Could you check a few things on this drawing? It's one solid part, dimensions in mm from its lowest x, y, z. A direction names the side the tool comes from. Round coordinates to 2 decimals unless told otherwise and drop trailing zeros. Loops run counter-clockwise (first coordinate to the right, second up) from the corner with the lowest first, then second, coordinate; pieces in that order, holes last. Notation, with made-up numbers: M 26,-1.75 L 31,-1.75 A11 ccw 31,7.25 Z; hole C 32.25,-27 d3. An arc over 180 degrees is marked long. Put each result on its own line as item: value. Start each with the question number.
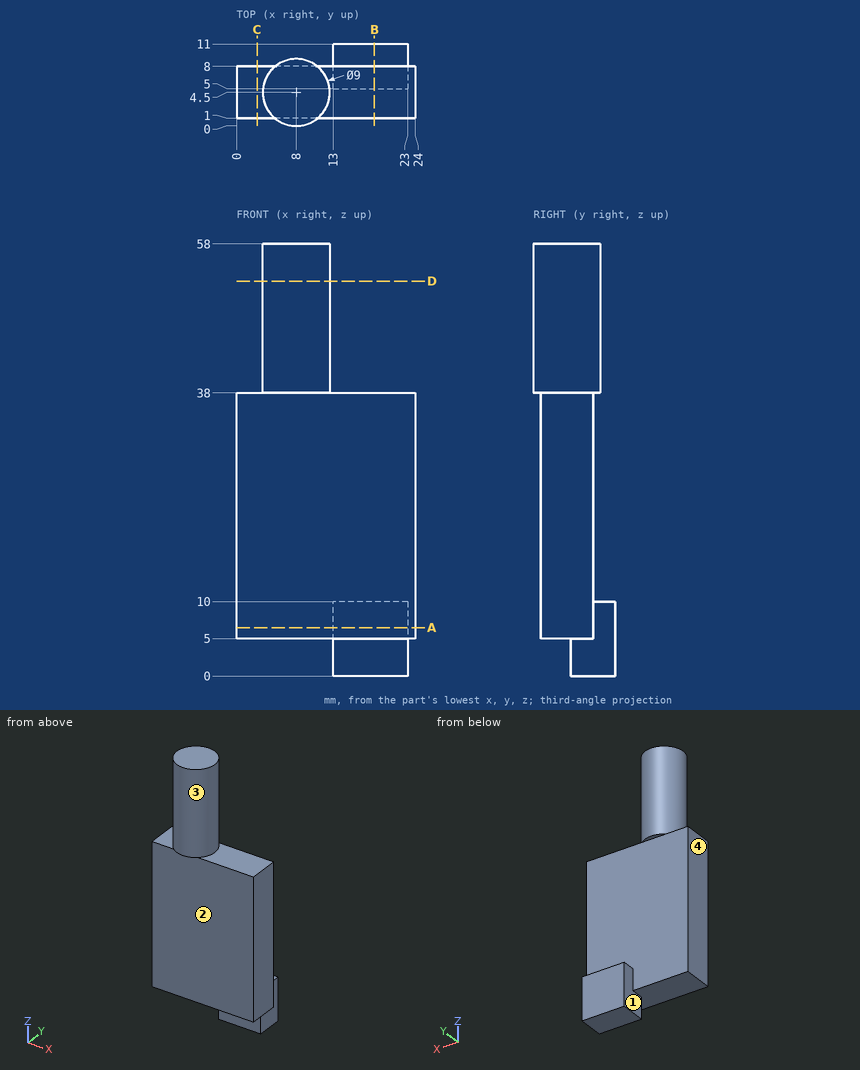
1) Suppose I cut it at C-C (x = 2.75). Write out the boundary of the cut face in (y, z).
2) Suppose I cut it at D-D (z = 53). Write out the boundary of the cut face in (x, y), plus the area to 3 significant figures.
3) Suppose I cut it at A-A (z = 6.5). Write out the boundary of the cut face in (x, y).
4) Suppose I cut it at B-B (x = 18.5). Write out the boundary of the cut face in (y, z), plus the area to 3 significant figures.
5) I'm going to push flat-ended pins straight in: P1, Ø4, axis at x = 19, z = 1.5, coming from the -Y side; P2, Ø3, axis at x = 14.5, y = 7.5, coming from the +Z side; P3, Ø4, axis at x = 5, z = 18, coming from the +Y side. Where does each tip first touch, or does it pass through?
6) On a 3-axis mill with a long thin cutter (end or side, diameter ignored), from which of +Z, -Z, +X, -X, +Y, -Y can I reach the whole of each face in a straight line? I mean the marked faces 1, 2, 3 and 4. Say none if no direction works.
7) If I drill on probe 1 along Z at (x, y) = (4.5, 4.75); probe 2 along Y at (x, z) = (14.25, 19); probe 3 along Z at (x, y) = (4, 7.5), over which ranges is the centre line in solid material (lowest first)? Write a range as from..to.
Results are:
1. outline: M 1,5 L 8,5 L 8,38 L 1,38 Z
2. outline: C 8,4.5 d9
2. area: 63.6 mm²
3. outline: M 0,1 L 24,1 L 24,8 L 23,8 L 23,11 L 13,11 L 13,8 L 0,8 Z
4. outline: M 1,5 L 5,5 L 5,0 L 11,0 L 11,10 L 8,10 L 8,38 L 1,38 Z
4. area: 276 mm²
5. P1: y = 5
5. P2: z = 38
5. P3: y = 8
6. face 1: -Z, -X, +Y
6. face 2: -Z, +X, -X, -Y
6. face 3: +Z
6. face 4: +Z, -Z, -X, +Y, -Y
7. probe 1: 5..58
7. probe 2: 1..8
7. probe 3: 5..38
